```python
from build123d import *

# Parameters (mm, degrees)
SKETCH_1_R          = 1.8
EXTRUDE_1_DEPTH     = 2
EXTRUDE_START       = -2
EXTRUDE_2_DEPTH     = 2
CUT_EXTRUDE_1_REACH = 58.535
SKETCH_4_R          = 1.5
CUT_EXTRUDE_2_REACH = 58.535
SKETCH_5_R          = 5


with BuildPart() as part:
    # 草图1 → 凸台-拉伸1 (new body)
    with BuildSketch(Plane.XY):
        with BuildLine():
            Line((-27.7, -32.7), (27.7, -32.7))
            ThreePointArc((27.7, -32.7), (31.235533906, -31.235533906), (32.7, -27.7))
            Line((32.7, -27.7), (32.7, 27.7))
            ThreePointArc((32.7, 27.7), (31.235533906, 31.235533906), (27.7, 32.7))
            Line((27.7, 32.7), (-27.7, 32.7))
            ThreePointArc((-27.7, 32.7), (-31.235533906, 31.235533906), (-32.7, 27.7))
            Line((-32.7, 27.7), (-32.7, -27.7))
            ThreePointArc((-32.7, -27.7), (-31.235533906, -31.235533906), (-27.7, -32.7))
        make_face()
        with Locations((24, 18)):
            Circle(SKETCH_1_R, mode=Mode.SUBTRACT)
        with Locations((-24, 18)):
            Circle(SKETCH_1_R, mode=Mode.SUBTRACT)
        with Locations((-24, -18)):
            Circle(SKETCH_1_R, mode=Mode.SUBTRACT)
        with Locations((24, -18)):
            Circle(SKETCH_1_R, mode=Mode.SUBTRACT)
    extrude(amount=EXTRUDE_1_DEPTH)

    # 草图3 → 凸台-拉伸2 (add)
    with BuildSketch(Plane.XY.offset(2).offset(EXTRUDE_START)):
        with BuildLine():
            Line((-39.951533137, 36.415999231), (-33.003300859, 29.467766953))
            Line((-33.003300859, 29.467766953), (-32.529629131, 28.994095226))
            ThreePointArc((-32.529629131, 28.994095226), (-31.235533906, 31.235533906), (-28.994095226, 32.529629131))
            Line((-28.994095226, 32.529629131), (-29.467766953, 33.003300859))
            Line((-29.467766953, 33.003300859), (-36.415999231, 39.951533137))
            Line((-36.415999231, 39.951533137), (-39.951533137, 36.415999231))
        make_face()
        with BuildLine():
            ThreePointArc((-28.994095226, 32.529629131), (-31.235533906, 31.235533906), (-32.529629131, 28.994095226))
            Line((-32.529629131, 28.994095226), (-31.037342597, 27.501808691))
            Line((-31.037342597, 27.501808691), (-27.501808691, 31.037342597))
            Line((-27.501808691, 31.037342597), (-28.994095226, 32.529629131))
        make_face()
        with BuildLine():
            ThreePointArc((32.529629131, 28.994095226), (31.235533906, 31.235533906), (28.994095226, 32.529629131))
            Line((28.994095226, 32.529629131), (27.501808691, 31.037342597))
            Line((27.501808691, 31.037342597), (31.037342597, 27.501808691))
            Line((31.037342597, 27.501808691), (32.529629131, 28.994095226))
        make_face()
        with BuildLine():
            Line((29.467766953, 33.003300859), (28.994095226, 32.529629131))
            ThreePointArc((28.994095226, 32.529629131), (31.235533906, 31.235533906), (32.529629131, 28.994095226))
            Line((32.529629131, 28.994095226), (33.003300859, 29.467766953))
            Line((33.003300859, 29.467766953), (39.951533137, 36.415999231))
            Line((39.951533137, 36.415999231), (36.415999231, 39.951533137))
            Line((36.415999231, 39.951533137), (29.467766953, 33.003300859))
        make_face()
        with BuildLine():
            Line((27.501808691, -31.037342597), (28.994095226, -32.529629131))
            ThreePointArc((28.994095226, -32.529629131), (31.235533906, -31.235533906), (32.529629131, -28.994095226))
            Line((32.529629131, -28.994095226), (31.037342597, -27.501808691))
            Line((31.037342597, -27.501808691), (27.501808691, -31.037342597))
        make_face()
        with BuildLine():
            ThreePointArc((32.529629131, -28.994095226), (31.235533906, -31.235533906), (28.994095226, -32.529629131))
            Line((28.994095226, -32.529629131), (29.467766953, -33.003300859))
            Line((29.467766953, -33.003300859), (36.415999231, -39.951533137))
            Line((36.415999231, -39.951533137), (39.951533137, -36.415999231))
            Line((39.951533137, -36.415999231), (33.003300859, -29.467766953))
            Line((33.003300859, -29.467766953), (32.529629131, -28.994095226))
        make_face()
        with BuildLine():
            ThreePointArc((-28.994095226, -32.529629131), (-31.235533906, -31.235533906), (-32.529629131, -28.994095226))
            Line((-32.529629131, -28.994095226), (-33.003300859, -29.467766953))
            Line((-33.003300859, -29.467766953), (-39.951533137, -36.415999231))
            Line((-39.951533137, -36.415999231), (-36.415999231, -39.951533137))
            Line((-36.415999231, -39.951533137), (-29.467766953, -33.003300859))
            Line((-29.467766953, -33.003300859), (-28.994095226, -32.529629131))
        make_face()
        with BuildLine():
            Line((-31.037342597, -27.501808691), (-32.529629131, -28.994095226))
            ThreePointArc((-32.529629131, -28.994095226), (-31.235533906, -31.235533906), (-28.994095226, -32.529629131))
            Line((-28.994095226, -32.529629131), (-27.501808691, -31.037342597))
            Line((-27.501808691, -31.037342597), (-31.037342597, -27.501808691))
        make_face()
    extrude(amount=EXTRUDE_2_DEPTH)

    # 草图4 → 切除-拉伸1 (cut, up to next)
    with BuildSketch(Plane.XY.offset(2), mode=Mode.PRIVATE) as cut_extrude_1_sk1:
        with Locations((-35.355339059, 35.355339059)):
            Circle(SKETCH_4_R)
    cut_extrude_1_tool1 = extrude(cut_extrude_1_sk1.sketch, amount=-CUT_EXTRUDE_1_REACH, mode=Mode.PRIVATE) & part.part
    # 草图4 → 切除-拉伸1 (cut, up to next)
    with BuildSketch(Plane.XY.offset(2), mode=Mode.PRIVATE) as cut_extrude_1_sk2:
        with Locations((35.355339059, 35.355339059)):
            Circle(SKETCH_4_R)
    cut_extrude_1_tool2 = extrude(cut_extrude_1_sk2.sketch, amount=-CUT_EXTRUDE_1_REACH, mode=Mode.PRIVATE) & part.part
    # 草图4 → 切除-拉伸1 (cut, up to next)
    with BuildSketch(Plane.XY.offset(2), mode=Mode.PRIVATE) as cut_extrude_1_sk3:
        with Locations((35.355339059, -35.355339059)):
            Circle(SKETCH_4_R)
    cut_extrude_1_tool3 = extrude(cut_extrude_1_sk3.sketch, amount=-CUT_EXTRUDE_1_REACH, mode=Mode.PRIVATE) & part.part
    # 草图4 → 切除-拉伸1 (cut, up to next)
    with BuildSketch(Plane.XY.offset(2), mode=Mode.PRIVATE) as cut_extrude_1_sk4:
        with Locations((-35.355339059, -35.355339059)):
            Circle(SKETCH_4_R)
    cut_extrude_1_tool4 = extrude(cut_extrude_1_sk4.sketch, amount=-CUT_EXTRUDE_1_REACH, mode=Mode.PRIVATE) & part.part
    add(cut_extrude_1_tool1.solids().sort_by_distance((-35.355339, 35.355339, 2))[0], mode=Mode.SUBTRACT)
    add(cut_extrude_1_tool2.solids().sort_by_distance((35.355339, 35.355339, 2))[0], mode=Mode.SUBTRACT)
    add(cut_extrude_1_tool3.solids().sort_by_distance((35.355339, -35.355339, 2))[0], mode=Mode.SUBTRACT)
    add(cut_extrude_1_tool4.solids().sort_by_distance((-35.355339, -35.355339, 2))[0], mode=Mode.SUBTRACT)

    # 草图5 → 切除-拉伸2 (cut, up to next)
    with BuildSketch(Plane.XY.offset(2), mode=Mode.PRIVATE) as cut_extrude_2_sk1:
        with Locations((-25.75, 0)):
            Circle(SKETCH_5_R)
    cut_extrude_2_tool1 = extrude(cut_extrude_2_sk1.sketch, amount=-CUT_EXTRUDE_2_REACH, mode=Mode.PRIVATE) & part.part
    # 草图5 → 切除-拉伸2 (cut, up to next)
    with BuildSketch(Plane.XY.offset(2), mode=Mode.PRIVATE) as cut_extrude_2_sk2:
        with Locations((12.875, 22.300154147)):
            Circle(SKETCH_5_R)
    cut_extrude_2_tool2 = extrude(cut_extrude_2_sk2.sketch, amount=-CUT_EXTRUDE_2_REACH, mode=Mode.PRIVATE) & part.part
    # 草图5 → 切除-拉伸2 (cut, up to next)
    with BuildSketch(Plane.XY.offset(2), mode=Mode.PRIVATE) as cut_extrude_2_sk3:
        with Locations((12.875, -22.300154147)):
            Circle(SKETCH_5_R)
    cut_extrude_2_tool3 = extrude(cut_extrude_2_sk3.sketch, amount=-CUT_EXTRUDE_2_REACH, mode=Mode.PRIVATE) & part.part
    add(cut_extrude_2_tool1.solids().sort_by_distance((-25.75, 0, 2))[0], mode=Mode.SUBTRACT)
    add(cut_extrude_2_tool2.solids().sort_by_distance((12.875, 22.300154, 2))[0], mode=Mode.SUBTRACT)
    add(cut_extrude_2_tool3.solids().sort_by_distance((12.875, -22.300154, 2))[0], mode=Mode.SUBTRACT)


solid = part.part
```
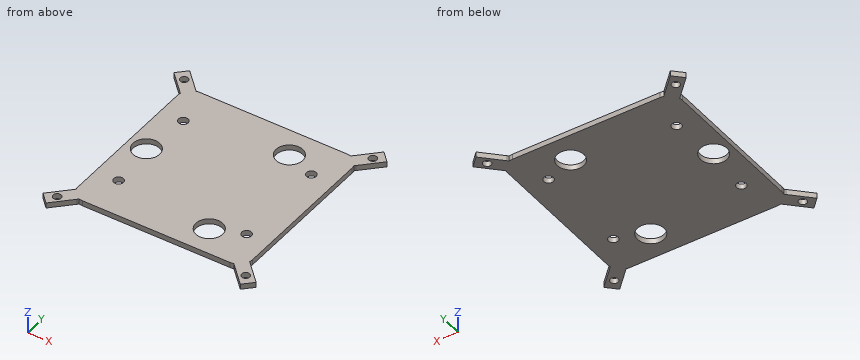
Input: part model. Units: mm. Frame: model coordinates. Round coordinates to 2 decimals unless told otherwise and drop trailing zeros. Write each loop counter-clockwise with the first axis right and the second up, starting at its lowest first coordinate (ties: lowest second). Pieces come first, ordered by that corner, then holes. Notation, with made-up numbers: (-15, 51) - (-2, 51) arc R13 cw to (-2, 73) - close; hole circle Ø2 at (78, 39). An arc over 180 degrees is marked (long way). Write item = value, one per line.
(1) Section query A-A on y = 0. Output: boundary loops of the cut face in (x, z).
Geometry check:
outline = (-32.7, 0) - (-30.75, 0) - (-30.75, 2) - (-32.7, 2) - close; (-20.75, 0) - (32.7, 0) - (32.7, 2) - (-20.75, 2) - close
(2) Section query D-D on x = -11. Output: boundary loops of the cut face in (y, z), then the cut area to 3 significant figures.
Geometry check:
outline = (-32.7, 0) - (32.7, 0) - (32.7, 2) - (-32.7, 2) - close
area = 131 mm^2
(3) Material intervals for probe 1 along Y at (x, z) = (24, 1.15); probe 2 along Y at (x, z) = (22, 1.1); probe 3 along X at (y, z) = (-35, 1.7), sorted ascending.
Geometry check:
probe_1 = -32.7 to -19.8, -16.2 to 16.2, 19.8 to 32.7
probe_2 = -32.7 to 32.7
probe_3 = -38.54 to -36.81, -33.9 to -31.46, 31.46 to 33.9, 36.81 to 38.54
(4) Section query B-B on x = 24. Output: boundary loops of the cut face in (y, z).
Geometry check:
outline = (-32.7, 0) - (-19.8, 0) - (-19.8, 2) - (-32.7, 2) - close; (-16.2, 0) - (16.2, 0) - (16.2, 2) - (-16.2, 2) - close; (19.8, 0) - (32.7, 0) - (32.7, 2) - (19.8, 2) - close
(5) Section query C-C on x = -24. Output: boundary loops of the cut face in (y, z).
Geometry check:
outline = (-32.7, 0) - (-19.8, 0) - (-19.8, 2) - (-32.7, 2) - close; (-16.2, 0) - (-4.68, 0) - (-4.68, 2) - (-16.2, 2) - close; (4.68, 0) - (16.2, 0) - (16.2, 2) - (4.68, 2) - close; (19.8, 0) - (32.7, 0) - (32.7, 2) - (19.8, 2) - close
(6) Contact query for flat-ended pins moving along their axis: pin 1 Ø1 at (y, z) = (-11.5, 1) entering from -X; pin 2 Ø0.6 at (y, z) = (-3.5, 1) entering from +X; pin 3 Ø2.5 at (x, y) = (35.36, -35.36) entering from -Z; pin 4 Ø1 at (x, z) = (25, 1.5) entering from +Y. Output: stop coordinate, or through.
Geometry check:
pin_1 = -32.7
pin_2 = 32.7
pin_3 = through
pin_4 = 32.7
